Geometry: final body of the model. Coordinates: model frame, mm. Face numbers are marked on the shaded views. A direction names the side the tool comes from. Round coordinates to 2 decimals unless told otherwise and drop trailing zeros. Loops run counter-clockwise (first coordinate to the right, second up) from the corner with the lowest first, then second, coordinate; pieces in that order, holes last. Notation, with made-up numbers: M -20.75,26 L -8.75,26 A32 ccw -8.75,59 Z; hole C 61.25,-37 d3. An arc over 180 degrees is marked long. Return JSON: item names as keys, results as strings.
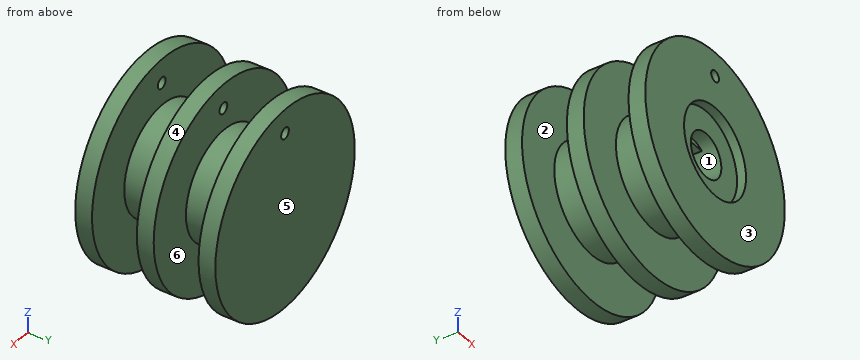
Autodesk Inventor part; units mm, degrees
ref_plane "YZ Plane" through (0, 0, 0) normal (1, 0, 0) x (0, 1, 0)
ref_plane "XZ Plane" through (0, 0, 0) normal (0, 1, 0) x (-1, 0, 0)
ref_plane "XY Plane" through (0, 0, 0) normal (0, 0, 1) x (1, 0, 0)
sketch "Sketch1" plane through (0, 0, 0) normal (0, 1, 0) x (-1, 0, 0)
  circle A0 centre (0, 0) radius 14.2875
  dimension "d0" = 28.575
extrude "Extrusion1" add sketch "Sketch1" along normal blind 2.3813
sketch "Sketch2" plane through (0, 2.3813, 0) normal (0, 1, 0) x (1, 0, 0)
  circle A0 centre (0, 0) radius 6.096 construction
  circle A1 centre (0, 0) radius 7.6835
  dimension "d6" = 12.192
  dimension "d7" = 1.5875
extrude "Extrusion2" add sketch "Sketch2" along normal blind 6.35
sketch "Sketch3" plane through (0, 8.7313, 0) normal (0, 1, 0) x (1, 0, 0)
  circle A0 centre (0, 0) radius 14.2875
  circle A1 centre (0, 0) radius 14.2875
extrude "Extrusion3" add sketch "Sketch3" along normal blind 2.3813
sketch "Sketch4" plane through (0, 11.1125, 0) normal (0, 1, 0) x (1, 0, 0)
  circle A0 centre (0, 0) radius 7.6835
  circle A1 centre (0, 0) radius 7.6835
extrude "Extrusion4" add sketch "Sketch4" along normal blind 6.35
sketch "Sketch5" plane through (0, 17.4625, 0) normal (0, 1, 0) x (1, 0, 0)
  circle A0 centre (0, 0) radius 14.2875
  circle A1 centre (0, 0) radius 14.2875
extrude "Extrusion5" add sketch "Sketch5" along normal blind 2.3813
sketch "Sketch6" plane through (0, 0, 0) normal (0, -1, 0) x (1, 0, 0)
  circle A0 centre (0, 0) radius 3.125
  line L0 (1.875, 2.5) -> (-1.875, 2.5)
  dimension "d16" = 6.25
  dimension "d35" = 2.5
extrude "Extrusion6" cut sketch "Sketch6" against normal through all contours A0 L0 picked at (0.5554, 0.5311)
sketch "Sketch7" plane through (0, 0, 0) normal (0, -1, 0) x (1, 0, 0)
  circle A0 centre (0, 0) radius 6.346
  dimension "d20" = 12.692
extrude "Extrusion7" cut sketch "Sketch7" against normal blind 1.27
sketch "Sketch8" plane through (0, 0, 0) normal (0, -1, 0) x (1, 0, 0)
  circle A0 centre (0, 0) radius 3.125
  arc A1 (-1.875, 2.5) -> (1.875, 2.5) centre (0, 0) ccw
extrude "Extrusion8" cut sketch "Sketch8" against normal blind 3.175
sketch "Sketch9" plane through (0, 19.8438, 0) normal (0, 1, 0) x (1, 0, 0)
  circle A0 centre (0, 0) radius 7.6835
  circle A1 centre (0, -10.8585) radius 0.7937
  point P0 (0, -7.6835)
  dimension "d31" = 1.5875
  dimension "d32" = 3.175
extrude "Extrusion9" cut sketch "Sketch9" against normal through all contours A1
sketch "Sketch10" plane through (0, 19.8438, 0) normal (0, 1, 0) x (1, 0, 0)
  circle A0 centre (0, -10.8585) radius 0.7937
  line L0 (1.875, -2.5) -> (-1.875, -2.5)
  arc A1 (1.875, -2.5) -> (-1.875, -2.5) centre (0, 0) ccw
  circle A2 centre (0, 0) radius 14.2875
extrude "Extrusion10" add sketch "Sketch10" against normal blind 5.842 contours L0 A1
equation "\"d10\" = d1"
equation "\"d12\" = d8"
equation "\"d14\" = d1"
equation "\"d18\" = d1"
properties part number "PulleyV2_3DPrint"
Q1. Pin query (flat end, axial travel): pin 1 (4.5 mm diameter, centred on x = 1, z = 0, fed in from -Y); pin 2 (4 mm diameter, centred on x = 4, y = 9, fed in from -Z); pin 3 (10 mm diameter, centred on y = 11.5, z = -7.5, fed in from +X). Return the tip coordinate at first contact, or that it passes through.
Determined:
{"pin 1": "stops at y = 1.27", "pin 2": "stops at z = -14.15", "pin 3": "stops at x = 14.06"}
Q2. Reachability of the marked faces 1, 2 and 3 from +Z, -Z, +X, -X, +Y, -Y: full face, straight path, thin tool, end or side. Return the list, or none.
Determined:
{"face 1": "-Y", "face 2": "none", "face 3": "+Z, -Z, +X, -X, -Y"}
Q3. Pull-direction query (Y, two-part tool) for the marked faces 4, 5 and 6; classes: pulls with the +Y half, pulls with the -Y half, needs draft (parallel to the pull), parting line crosses it, or undercut.
Determined:
{"face 4": "needs draft", "face 5": "pulls with the +Y half", "face 6": "undercut"}
Q4. Section query C-C (z = -9.75). Output: boundary loops of the cut face in (x, y).
Determined:
{"outline": "M -10.44,0 L 10.44,0 L 10.44,2.38 L -10.44,2.38 Z; M -10.44,8.73 L 10.44,8.73 L 10.44,11.11 L -10.44,11.11 Z; M -10.44,17.46 L 10.44,17.46 L 10.44,19.84 L -10.44,19.84 Z"}
Q5. Section query B-B (x = 11.75). Output: boundary loops of the cut face in (y, z), plus the area to 3 significant figures.
Determined:
{"outline": "M 0,-8.13 L 2.38,-8.13 L 2.38,8.13 L 0,8.13 Z; M 8.73,-8.13 L 11.11,-8.13 L 11.11,8.13 L 8.73,8.13 Z; M 17.46,-8.13 L 19.84,-8.13 L 19.84,8.13 L 17.46,8.13 Z", "area": "116 mm^2"}
Q6. Material intervals for L1, parallel to Z at x = 0, y = 9.75 (1 decimal); L2, parallel to Y at x = -8.25, z = -1.5; L3, parallel to X at y = 11.5, z = 0 (1 decimal), sorted ascending.
Determined:
{"L1": "z = -14.3 to -3.1, 2.5 to 10.1, 11.7 to 14.3", "L2": "y = 0 to 2.38, 8.73 to 11.11, 17.46 to 19.84", "L3": "x = -7.7 to -3.1, 3.1 to 7.7"}
Q7. Section query A-A (z = 0). Output: boundary loops of the cut face in (x, y) (1 decimal), plus the area to 3 significant figures.
Determined:
{"outline": "M -14.3,0 L -6.3,0 L -6.3,1.3 L -3.1,1.3 L -3.1,14 L 3.1,14 L 3.1,1.3 L 6.3,1.3 L 6.3,0 L 14.3,0 L 14.3,2.4 L 7.7,2.4 L 7.7,8.7 L 14.3,8.7 L 14.3,11.1 L 7.7,11.1 L 7.7,17.5 L 14.3,17.5 L 14.3,19.8 L -14.3,19.8 L -14.3,17.5 L -7.7,17.5 L -7.7,11.1 L -14.3,11.1 L -14.3,8.7 L -7.7,8.7 L -7.7,2.4 L -14.3,2.4 Z", "area": "304 mm^2"}
